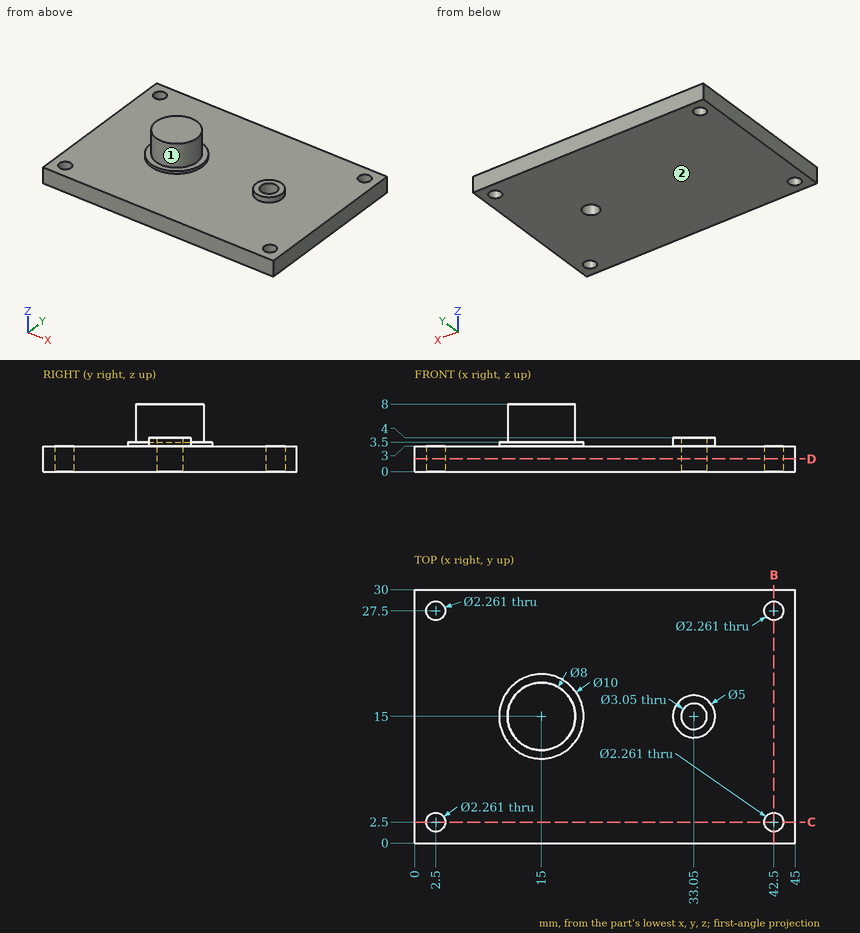
Part print with two shaded views. Sizes in mm from the minimum x, y, z corner. A direction names the side the tool comes from. Round coordinates to 2 decimals unless told otherwise and drop trailing zeros. Loops run counter-clockwise (first coordinate to the right, second up) from the corner with the lowest first, then second, coordinate; pieces in that order, holes last. Notation, with made-up numbers: (85, 69.5) - (113, 69.5) arc R23 cw to (113, 103.5) - close; hole circle Ø4 at (16, -38). An arc over 180 degrees is marked (long way). Put each result on its own line as item: value.
1. Slice it at D-D on z = 1.5. Give the number of separate pieces and of enclosed holes in the cut face, and give its area (3 significant figures).
Geometry check:
separate pieces: 1
enclosed holes: 5
area: 1,330 mm²
2. 3-axis set-ups, long thin cutter, end or side, ignore diameter. For the marked faces 1 and 2: which of +Z, -Z, +X, -X, +Y, -Y reach the whole face in a straight line?
Geometry check:
face 1: +Z
face 2: -Z, +X, -X, +Y, -Y
3. Pin check, flat tips, straight feed: P1, Ø2, axis at x = 42.5, y = 27.5, coming from the +Z side; P2, Ø1, axis at x = 26.5, y = 20.5, coming from the +Z side; P3, Ø5.5, axis at x = 33.5, y = 14, coming from the +Z side. Stop position of each tip, or through.
Geometry check:
P1: through
P2: z = 3
P3: z = 4
4. Slice it at B-B on x = 42.5. List the corners of the cut face in (y, z).
Geometry check:
outline: (0, 0) - (1.37, 0) - (1.37, 3) - (0, 3) - close; (3.63, 0) - (26.37, 0) - (26.37, 3) - (3.63, 3) - close; (28.63, 0) - (30, 0) - (30, 3) - (28.63, 3) - close
5. Slice it at C-C on y = 2.5. List the corners of the cut face in (x, z).
Geometry check:
outline: (0, 0) - (1.37, 0) - (1.37, 3) - (0, 3) - close; (3.63, 0) - (41.37, 0) - (41.37, 3) - (3.63, 3) - close; (43.63, 0) - (45, 0) - (45, 3) - (43.63, 3) - close
6. Wall check: line 1 (Y direction, x = 42.5, z = 1.65); line 2 (Z direction, x = 40, y = 4.75); line 3 (X direction, y = 15.5, z = 2.75). Give the ranges that are in metal, low to high.
Geometry check:
line 1: 0 to 1.37, 3.63 to 26.37, 28.63 to 30
line 2: 0 to 3
line 3: 0 to 31.61, 34.49 to 45
